For this review, take the finished solid that the model builds, in its own axes (mm). A direction names the side the tool comes from. Give positions to 0.01 mm unless a question says otherwise; leave off trailing zeros. Write each loop counter-clockwise with the first axis right and the second up, starting at its lowest first coordinate (ties: lowest second). Pieces come first, ordered by that corner, then holes.
from build123d import *

# Parameters (mm, degrees)
F1_DEPTH = 25.4
F2_W     = 52.48428
F2_H     = 6.35
F3_DEPTH = 6.35
F4_W     = 52.48428
F4_H     = 6.35
F5_DEPTH = 6.35


with BuildPart() as f1:
    # F0 (on Front) → F1 (new body)
    with BuildSketch(Plane.XZ):
        Polygon((4.563851, 37.509143), (4.563851, 0), (22.248767, 0), (22.248767, 9.840802), (38.792729, 9.840802), (38.792729, 0), (57.048131, 0), (57.048131, 37.509143), align=None)
    extrude(amount=F1_DEPTH)

    # F2 (on face) → F3 (join)
    with BuildSketch(Plane.XY.offset(37.509143)):
        with Locations((30.805991, -3.175)):
            Rectangle(F2_W, F2_H)
    extrude(amount=F3_DEPTH)

    # F4 (on face) → F5 (join)
    with BuildSketch(Plane.XY.offset(37.509143)):
        with Locations((30.805991, -22.225)):
            Rectangle(F4_W, F4_H)
    extrude(amount=F5_DEPTH)


solid = f1.part
(1) We need section A-A (y = -15.25). Write out the cut boundary in (x, z), and give its area (3 significant figures).
(2) The part is to be moulded in two halves that separate along Y. For faces 4 (the flat face through (30, -19.05, 41)), 5 (the flat face through (31, -13, 37.509)), 6 (the flat face through (22.249, -13, 5)), 7 (the flat face through (30, 0, 22)), say which applies: +Y half, -Y half, draft (parallel to the pull), parting line (faces both ways), or undercut.
(3) Tool access review of faces 1 (the flat face through (30, -25.4, 22)), 2 (the flat face through (30, -6.35, 41)), 3 (the flat face through (30, -13, 9.841)): name each direction out of +Z, -Z, +X, -X, +Y, -Y from which nothing blocks a thin tool from reaching the whole face with its end or side.
(4) Clearance check with flat-ended pins moving along their axes: pin 1 Ø2 at (x, y) = (30, -12.5) entering from +Z; pin 2 Ø2 at (x, y) = (34.5, -17) entering from -Z. State where each tip first meets the part, or that it passes through.
(5) We need section B-B (x = 16). Write out the cut boundary in (y, z), and give its area (3 significant figures).
(6) For L1, parallel to X at y = -3, z = 3; L2, parallel to Y at x = 23, z = 41; L3, parallel to Z at x = 14.5, y = -17, list the stretches that pass through material, from the lowest coordinate up.
The answers:
1. outline: (4.56, 0) - (22.25, 0) - (22.25, 9.84) - (38.79, 9.84) - (38.79, 0) - (57.05, 0) - (57.05, 37.51) - (4.56, 37.51) - close
1. area: 1,810 mm2
2. face 4: undercut
2. face 5: undercut
2. face 6: draft
2. face 7: +Y half
3. face 1: +Z, -Z, +X, -X, -Y
3. face 2: +Z, +X, -X
3. face 3: -Z, +Y, -Y
4. pin 1: stops at z = 37.51
4. pin 2: stops at z = 9.84
5. outline: (-25.4, 0) - (0, 0) - (0, 43.86) - (-6.35, 43.86) - (-6.35, 37.51) - (-19.05, 37.51) - (-19.05, 43.86) - (-25.4, 43.86) - close
5. area: 1,030 mm2
6. L1: x = 4.56 to 22.25, 38.79 to 57.05
6. L2: y = -25.4 to -19.05, -6.35 to 0
6. L3: z = 0 to 37.51
